Model file for the job. Use its own axes, mm. A direction names the side the tool comes from. Coordinates: 2 decimals unless noted, no trailing zeros. Order: outer loops, then holes, each group sorted by start corner. A loop starts at its lowest first (then second) coordinate and runs counter-clockwise, first axis right, second up. Notation, with made-up numbers: (80, 58.25) -> (116, 58.25) arc R14 ccw to (116, 62.25) -> close; hole circle Ø11 at (-39.5, -24.75). An arc over 180 degrees is marked (long way). Write item = value, one per line. Start each with the question number.
Q1. 3-axis set-ups, long thin cutter, end or side, ignore diameter. For faces 4 (the face through (65, 2, -11)), 5 (the face through (64.1, 4, -29.2)): which of +Z, -Z, +X, -X, +Y, -Y reach the whole face in a straight line?
Q2. Cut at D-D, the plane y = 2.5. Give the number of separate pieces and of enclosed holes in the cut face, plus the area to 3 significant figures.
Q3. Cut at B-B, the plane z = -35. List the corners of the cut face in (x, y).
Q4. Cut at C-C, the plane x = 25.5. List the corners of the cut face in (y, z), plus the area to 3 significant figures.
Q5. Flat gauge pins, fed straight in: pin 1 (5 mm diameter, centred on x = 120.5, z = -35, fed in from -Y); pin 2 (4 mm diameter, centred on x = 120.5, z = -5, fed in from -Y). Where does each tip first touch, or does it go through?
Q6. Cut at A-A, the plane x = 9.5. List the corners of the cut face in (y, z), plus the area to 3 significant figures.
Q7. Mould opens along Z. For faces 1 (the face through (45.16, 2.76, -35.85)), 2 (the face through (64.1, 0, -29.2)), 3 (the face through (64, 2, 0)) say: +Z half, -Z half, draft (parallel to the pull), parting line (faces both ways), or undercut.
Q8. Wall check: line 1 (Z direction, x = 120.5, y = 2.2); line 2 (Z direction, x = 83.5, y = 2.2); line 3 (X direction, y = 3.45, z = -35). Give the ranges that are in metal, low to high. Write a range as from..to.
from build123d import *

# Parameters (mm, degrees)
ESBO_O1_W                 = 130
ESBO_O1_H                 = 40
RESSALTO_EXTRUS_O1_DEPTH  = 4
PADR_O_LINEAR1_COUNT      = 4
PADR_O_LINEAR1_PITCH      = 37
PADR_O_LINEAR1_COUNT_DIR2 = 2
PADR_O_LINEAR1_PITCH_DIR2 = 30


with BuildPart() as part:
    # Esboço1 → Ressalto-extrusão1 (new body)
    with BuildSketch(Plane(origin=(0, 0, 0), x_dir=(1, 0, 0), z_dir=(0, 1, 0))):
        with Locations((65, 20)):
            Rectangle(ESBO_O1_W, ESBO_O1_H)
        with BuildLine():
            Line((22, 29), (106, 29))
            ThreePointArc((106, 29), (115, 20), (106, 11))
            Line((106, 11), (22, 11))
            ThreePointArc((22, 11), (13, 20), (22, 29))
        make_face(mode=Mode.SUBTRACT)
    extrude(amount=RESSALTO_EXTRUS_O1_DEPTH)

    # Esboço4 → Escareado para parafuso com cabeça escareada elevada de M31 (revolve, cut)
    with BuildSketch(Plane(origin=(9.5, 0, -35), x_dir=(0, 0, -1), z_dir=(1, 0, 0))):
        Polygon((0, 0), (0, 13.953866233), (1.5875, 13), (1.5875, 1.5625), (3.15, 0), align=None)
    escareado_para_parafuso_com_cabe_a_escar = revolve(axis=Axis((9.5, -6.35, -35), (0, 1, 0)), mode=Mode.SUBTRACT)

    # Padrão linear1: Escareado para parafuso com cabe_a escar 4 × 2
    with Locations(*[(i * PADR_O_LINEAR1_PITCH, 0, j * PADR_O_LINEAR1_PITCH_DIR2) for i in range(PADR_O_LINEAR1_COUNT) for j in range(PADR_O_LINEAR1_COUNT_DIR2) if (i, j) != (0, 0)]):
        add(escareado_para_parafuso_com_cabe_a_escar, mode=Mode.SUBTRACT)


solid = part.part
Here are the results:
q1.face_4 = +Y, -Y
q1.face_5 = +Z, -Z, +X, -X, +Y
q2.separate_pieces = 1
q2.enclosed_holes = 9
q2.area = 3,370 mm²
q3.outline = (0, 0) -> (6.35, 0) -> (7.91, 1.56) -> (7.91, 4) -> (0, 4) -> close; (11.09, 1.56) -> (12.65, 0) -> (43.35, 0) -> (44.91, 1.56) -> (44.91, 4) -> (11.09, 4) -> close; (48.09, 1.56) -> (49.65, 0) -> (80.35, 0) -> (81.91, 1.56) -> (81.91, 4) -> (48.09, 4) -> close; (85.09, 1.56) -> (86.65, 0) -> (117.35, 0) -> (118.91, 1.56) -> (118.91, 4) -> (85.09, 4) -> close; (122.09, 1.56) -> (123.65, 0) -> (130, 0) -> (130, 4) -> (122.09, 4) -> close
q4.outline = (0, -40) -> (4, -40) -> (4, -29) -> (0, -29) -> close; (0, -11) -> (4, -11) -> (4, 0) -> (0, 0) -> close
q4.area = 88.0 mm²
q5.pin_1 = 0.65
q5.pin_2 = 1.15
q6.outline = (0, -40) -> (4, -40) -> (4, -36.59) -> (1.56, -36.59) -> (0, -38.15) -> close; (0, -31.85) -> (1.56, -33.41) -> (4, -33.41) -> (4, -6.59) -> (1.56, -6.59) -> (0, -8.15) -> close; (0, -1.85) -> (1.56, -3.41) -> (4, -3.41) -> (4, 0) -> (0, 0) -> close
q6.area = 130 mm²
q7.face_1 = undercut
q7.face_2 = draft
q7.face_3 = +Z half
q8.line_1 = -40..-36.59, -33.41..-6.59, -3.41..0
q8.line_2 = -40..-36.59, -33.41..-29, -11..-6.59, -3.41..0
q8.line_3 = 0..7.91, 11.09..44.91, 48.09..81.91, 85.09..118.91, 122.09..130
